from build123d import *

# Parameters (mm, degrees)
SKETCH2_R          = 2
SKETCH3_W          = 22
SKETCH3_H          = 22
CUT_EXTRUDE1_DEPTH = 2934.581386125


with BuildPart() as part:
    # Sweep1: sweep along a path in Sketch1
    with BuildLine(Plane.XY) as sweep1_path:
        Line((0, 0), (0, 1670))
        ThreePointArc((0, 1670), (83.474567362, 1871.525432638), (285, 1955))
        Line((285, 1955), (1845, 1955))
        ThreePointArc((1845, 1955), (2046.525432638, 1871.525432638), (2130, 1670))
        Line((2130, 1670), (2130, 0))
    # Sketch2 → Sweep1 (sweep)
    with BuildSketch(Plane(origin=(0, 0, 0), x_dir=(1, 0, 0), z_dir=(0, 1, 0))):
        with BuildLine():
            Line((0, 0), (0, -2))
            ThreePointArc((0, -2), (-3, -8.645751311), (-6, -2))
            Line((-6, -2), (-30, -2))
            Line((-30, -2), (-30, 0))
            Line((-30, 0), (0, 0))
        make_face()
        with Locations((-3, -4.645751311)):
            Circle(SKETCH2_R, mode=Mode.SUBTRACT)
    sweep(path=sweep1_path.line)

    # Sketch3 → Cut-Extrude1 (cut, through all)
    with BuildSketch(Plane(origin=(0, 0, 0), x_dir=(-1, 0, 0), z_dir=(0, 0, -1))):
        with Locations((-1415, 1970)):
            Rectangle(SKETCH3_W, SKETCH3_H)
        with Locations((-715, 1970)):
            Rectangle(SKETCH3_W, SKETCH3_H)
    extrude(amount=-CUT_EXTRUDE1_DEPTH, mode=Mode.SUBTRACT)


solid = part.part
Input: part model. Units: mm. Frame: model coordinates. Coordinates: 2 decimals unless noted, no trailing zeros. Loops run counter-clockwise (first coordinate to the right, second up) from the corner with the lowest first, then second, coordinate; pieces in that order, holes last.
(1) Section A-A on y = 675. Return the cut outline in (x, z).
(2) Material intervals for probe 1 along X at (y, z) = (1443.5, 5); probe 2 along X at (y, z) = (201, 3.25); probe 3 along X at (y, z) = (923, 1.5), sorted ascending.
(3) Pull-direction query (X, two-part tool) for faces 1 (the face through (81.271, 1869.297, 0.986)), 2 (the face through (2065.28, 1895.17, 1.01)), 3 (the face through (59.83, 1890.28, 1.01)); classes: released by +X, released by -X, zero draft, split by the parting line, or undercut.
(4) Section B-B on x = 354.5. Return the cut outline in (y, z).
(5) Section C-C on y = 1805. Count the separate pieces of the cut face and the enclosed holes in it, then the cut area to 3 significant figures.
(6) First-contact query: pin 1 Ø1.6 at (x, z) = (1211, 1) entering from -Y; pin 2 Ø1 at (x, z) = (485, 7.5) entering from +Y; pin 3 Ø5 at (x, z) = (1887, 3) entering from +Y; pin 4 Ø5 at (x, z) = (-3, 4.65) entering from -Y. Flat tips, straight axial feed; report the tip coordinate or a pass-through.
Data:
1. outline: (-30, 0) - (0, 0) - (0, 2) arc R4 ccw (long way) to (-6, 2) - (-30, 2) - close; (2130, 0) - (2160, 0) - (2160, 2) - (2136, 2) arc R4 ccw (long way) to (2130, 2) - close; hole circle Ø4 at (-3, 4.65); hole circle Ø4 at (2133, 4.65)
2. probe 1: x = -6.98 to -4.97, -1.03 to 0.98, 2129.02 to 2131.03, 2134.97 to 2136.98
2. probe 2: x = -6.75 to -4.43, -1.57 to 0.75, 2129.25 to 2131.57, 2134.43 to 2136.75
2. probe 3: x = -30 to 0, 2130 to 2160
3. face 1: undercut
3. face 2: released by +X
3. face 3: released by -X
4. outline: (1955, 0) - (1985, 0) - (1985, 2) - (1961, 2) arc R4 ccw (long way) to (1955, 2) - close; hole circle Ø4 at (1958, 4.65)
5. separate pieces: 2
5. enclosed holes: 2
5. area: 207 mm2
6. pin 1: stops at y = 1955
6. pin 2: stops at y = 1961.23
6. pin 3: stops at y = 1982.49
6. pin 4: stops at y = 0
